from build123d import *

# Parameters (mm, degrees)
F1_DEPTH = 63.5
F2_DEPTH = 38.1
F3_DEPTH = 12.7
F5_R     = 5.08


with BuildPart() as f1:
    # F0 (on Front) → F1 (new body, symmetric)
    with BuildSketch(Plane.XZ):
        Polygon((-38.1, -12.7), (38.1, -12.7), (38.1, 12.7), (19.05, 12.7), (-38.1, 12.7), align=None)
    extrude(amount=F1_DEPTH, both=True)

    # F0 (on Front) → F2 (join, symmetric)
    with BuildSketch(Plane.XZ):
        with BuildLine():
            Line((19.05, 12.7), (38.1, 12.7))
            Line((38.1, 12.7), (38.1, 28.2195249445))
            ThreePointArc((38.1, 28.2195249445), (40.2827686763, 34.511534195), (45.8931851198, 38.1))
            Line((45.8931851198, 38.1), (57.15, 38.1))
            Line((57.15, 38.1), (57.15, 57.15))
            Line((57.15, 57.15), (44.2286586523, 57.15))
            ThreePointArc((44.2286586523, 57.15), (26.2261671427, 47.395924753), (19.05, 28.2195249445))
            Line((19.05, 28.2195249445), (19.05, 12.7))
        make_face()
        Polygon((82.5615462799, 57.15), (57.15, 57.15), (57.15, 38.1), (82.5961851198, 38.1), align=None)
    extrude(amount=F2_DEPTH, both=True)

    # F0 (on Front) → F3 (join, symmetric)
    with BuildSketch(Plane.XZ):
        with BuildLine():
            add(Edge.make_bspline(
                [(-38.1, 12.7), (-33.8629931211, 55.5353052914), (0, 61.6306401789), (57.15, 63.5)],
                knots=[0, 0, 0, 0, 107.95, 107.95, 107.95, 107.95], degree=3))
            Line((-38.1, 12.7), (19.05, 12.7))
            Line((19.05, 12.7), (19.05, 28.2195249445))
            ThreePointArc((19.05, 28.2195249445), (26.2261671427, 47.395924753), (44.2286586523, 57.15))
            Line((44.2286586523, 57.15), (57.15, 57.15))
            Line((57.15, 57.15), (57.15, 63.5))
        make_face()
    extrude(amount=F3_DEPTH, both=True)

    # F0 (on Front) → F4 (revolve)
    with BuildSketch(Plane.XZ):
        Polygon((107.95, 63.5), (82.55, 63.5), (82.5615462799, 57.15), (82.5961851198, 38.1), (107.95, 38.1), align=None)
    revolve(axis=Axis((82.5730925599, 0, 50.8), (0.0018183088, 0, -0.9999983469)))

    # F5
    f5_edges = [f1.edges().sort_by_distance(p)[0] for p in [
        (38.1, -63.5, 0),
        (-38.1, -63.5, 0),
        (38.1, 63.5, 0),
        (-38.1, 63.5, 0),
    ]]
    fillet(f5_edges, radius=F5_R)


solid = f1.part
Read the model definition and answer for the solid it produces. Units are mm, in the model's axes. A direction names the side the tool comes from. Give positions to 0.01 mm unless a question says otherwise; leave off trailing zeros. Write each loop counter-clockwise with the first axis right and the second up, starting at its lowest first coordinate (ties: lowest second). Pieces come first, ordered by that corner, then holes. Notation, with made-up numbers: (-26, 78) - (1, 78) arc R27 ccw to (1, 110) - close; hole circle Ø7 at (44, 85). An arc over 180 degrees is marked (long way). Answer in a Markdown table with one row per item. Add a question column.
Item 1: Section A-A, the plane y = 28.5 is taken. Write down the section's boundary in (x, z), and give its area (3 significant figures).
Item 2: Section B-B, the plane z = 7.5 is taken. Write down the section's boundary in (x, y), and give its area (3 significant figures).
Item 3: Flat-ended cylindrical pins translate along their axes: P1, Ø1, axis at x = -4.5, z = 47.5, coming from the +Y side; P2, Ø5, axis at x = 10, y = 2.5, coming from the +Z side; P3, Ø12.5, axis at y = -31, z = 22, coming from the -X side. Find the tip coordinate at first contact, or state that the pin passes through.
Item 4: Section C-C, the plane y = 52 is taken. Write down the section's boundary in (x, z).
Item 5: A tool of negligible diameter and unlimited length cuts with its end or side. For faces 1 (the face through (26.42, -25.578, 47.616)), 2 (the face through (26.42, 25.222, 47.616)), from which of +Z, -Z, +X, -X, +Y, -Y can it reach the whole face along a straight path? Write none if from no direction.
Item 6: Find the intervals of material crossed by L1, parallel to X at y = 22, z = 17; L2, parallel to Z at x = -9, y = -56; L3, parallel to Z at x = 89.5, y = 23.5, in increasing order.
Recorded:
| question | item | result |
|---|---|---|
| 1 | outline | (-38.1, -12.7) - (38.1, -12.7) - (38.1, 28.22) arc R10.16 cw to (45.89, 38.1) - (82.6, 38.1) - (82.56, 57.15) - (44.23, 57.15) arc R29.21 ccw to (19.05, 28.22) - (19.05, 12.7) - (-38.1, 12.7) - close |
| 1 | area | 3,470 mm2 |
| 2 | outline | (-38.1, -58.42) arc R5.08 ccw to (-33.02, -63.5) - (33.02, -63.5) arc R5.08 ccw to (38.1, -58.42) - (38.1, 58.42) arc R5.08 ccw to (33.02, 63.5) - (-33.02, 63.5) arc R5.08 ccw to (-38.1, 58.42) - close |
| 2 | area | 9,660 mm2 |
| 3 | P1 | stops at y = 12.7 |
| 3 | P2 | stops at z = 59.85 |
| 3 | P3 | stops at x = 19.05 |
| 4 | outline | (-38.1, -12.7) - (38.1, -12.7) - (38.1, 12.7) - (-38.1, 12.7) - close |
| 5 | face 1 | +Z, -X, -Y |
| 5 | face 2 | +Z, -X, +Y |
| 6 | L1 | x = 19.05 to 38.1 |
| 6 | L2 | z = -12.7 to 12.7 |
| 6 | L3 | z = 38.07 to 63.47 |
